from build123d import *

# Parameters (mm, degrees)
F0_W     = 344
F0_H     = 364
F1_DEPTH = 400
F2_T     = -2
F4_START = -25
F4_DEPTH = 319.001


with BuildPart() as f1:
    # F0 (on Front) → F1 (new body)
    with BuildSketch(Plane.XZ):
        with Locations((172, -182)):
            Rectangle(F0_W, F0_H)
    extrude(amount=F1_DEPTH)

    # F2
    f2_openings = [f1.faces().sort_by_distance(p)[0] for p in [
        (172, -200, 0),
    ]]
    offset(amount=F2_T, openings=f2_openings)

    # F3 (on face) → F4 (cut)
    with BuildSketch(Plane.YZ.offset(344).offset(F4_START)):
        with BuildLine():
            Line((-380.2282512188, -42.8705103695), (-380.2282512188, -279.8911333084))
            add(Edge.make_bspline(
                [(-380.2282512188, -279.8911333084), (-335.3109516688, -297.4034551854), (-244.5381641795, -332.7938791003), (-101.0842446911, -244.1373138208), (-46.4290637673, -287.7654343562), (-22.6302593946, -306.7626655102)],
                knots=[0, 0, 0, 0, 0.3560906868, 0.7196190458, 1, 1, 1, 1], degree=3))
            Line((-22.6302593946, -306.7626655102), (-22.6302593946, -42.8705103695))
            Line((-22.6302593946, -42.8705103695), (-380.2282512188, -42.8705103695))
        make_face()
    extrude(amount=-F4_DEPTH, mode=Mode.SUBTRACT)


solid = f1.part
Work out the finished part from the listing and answer in its coordinate system (mm). A direction names the side the tool comes from. Give positions to 0.01 mm unless a question says otherwise; leave off trailing zeros. Loops run counter-clockwise (first coordinate to the right, second up) from the corner with the lowest first, then second, coordinate; pieces in that order, holes last. Notation, with made-up numbers: M 81,27 L 110,27 A15 ccw 110,32 Z; hole C 45.5,4 d8. An arc over 180 degrees is marked long. Use CSV: the item, a comma, the result in double quotes.
1) Find section B-B on x = 64. Write down the section's boundary in (y, z), plus the area to 3 significant figures.
Answer:
outline,"M -400,-364 L 0,-364 L 0,0 L -2,0 L -2,-362 L -398,-362 L -398,0 L -400,0 Z"
area,"2,250 mm^2"
2) Consider L1, parallel to Y at x = 227.5, z = -341; L2, parallel to X at y = -285, z = -75; L3, parallel to Z at x = 118, y = -85. Determine where each line is inside the solid, lowest interval first.
Answer:
L1,"-400 to -398, -2 to 0"
L2,"342 to 344"
L3,"-364 to -362"
3) Find section C-C on z = -101. Write down the section's boundary in (x, y), plus the area to 3 significant figures.
Answer:
outline,"M 0,-400 L 344,-400 L 344,0 L 0,0 L 0,-22.63 L 2,-22.63 L 2,-2 L 342,-2 L 342,-398 L 2,-398 L 2,-380.23 L 0,-380.23 Z"
area,"2,240 mm^2"
4) Determine the mould class of faces 3 (the flat face through (170, -400, -179)), 4 (the flat face through (170, -197, -362)), 5 (the flat face through (344, -197, -185)) for opening direction Y: released by +Y, released by -Y, zero draft, split by the parting line, or undercut.
Answer:
face 3,"released by -Y"
face 4,"undercut"
face 5,"zero draft"
5) Which of the six approach directions +Z, -Z, +X, -X, +Y, -Y give full straight-line access (tool end or side, diameter ignored) to faces 1 (the flat face through (170, -197, -364)), 2 (the flat face through (170, -398, -178))?
Answer:
face 1,"-Z, +X, -X, +Y, -Y"
face 2,"+Z"
6) Find section A-A on z = -332.5. Write down the section's boundary in (x, y), plus the area to 3 significant figures.
Answer:
outline,"M 0,-400 L 344,-400 L 344,0 L 0,0 Z; hole M 2,-398 L 342,-398 L 342,-2 L 2,-2 Z"
area,"2,960 mm^2"
7) Given P1, Ø10, axis at x = 282, z = -182.5, coming from the +Y side; P2, Ø1.5, axis at y = -57.5, z = -96.5, coming from the -X side; P3, Ø6, axis at x = 249.5, y = -228.5, coming from the +Z side, each flat-ended and moving along its own axis, determine where each tip first touches the part or whether it passes through.
Answer:
P1,"y = 0"
P2,"x = 342"
P3,"z = -362"
